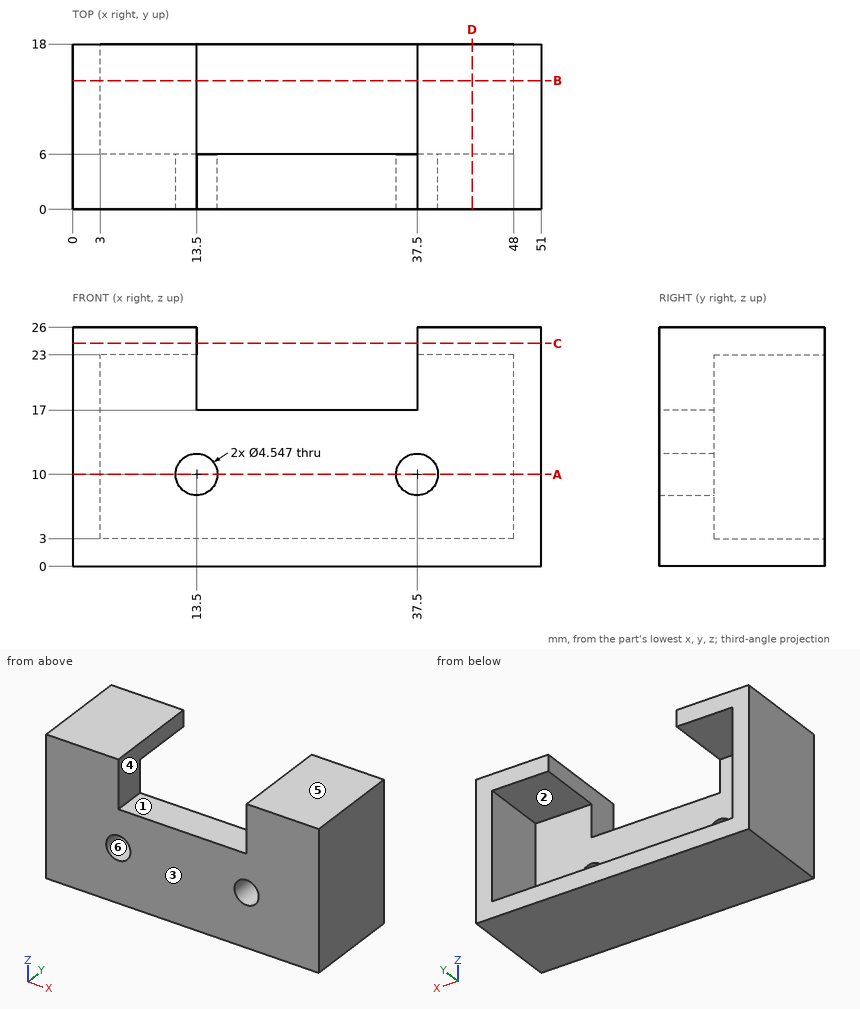
Design review of the part shown in the three views and the two pictorial views. Dimensions are in mm from the part's minimum x, y and z. A direction names the side the tool comes from. Coordinates: 2 decimals unless noted, no trailing zeros. Order: outer loops, then holes, each group sorted by start corner. A loop starts at its lowest first (then second) coordinate and runs counter-clockwise, first axis right, second up. Notation, with made-up numbers: (-6, 46) -> (7, 46) arc R24 cw to (7, 85) -> close; hole circle Ø2 at (18.25, -33). An arc over 180 degrees is marked (long way). Use one line per item in the form item = value. Start each with the question number.
(1) For probe 1 along X at (y, z) = (3.5, 10); probe 2 along X at (y, z) = (9, 8.5); probe 3 along Z at (x, y) = (10.5, 15), list the stretches that pass through material, from the lowest coordinate up.
(2) The part is to be moulded in two halves that separate along Z. For the marked faces 4, 5 and 6, say which applies: +Z half, -Z half, draft (parallel to the pull), parting line (faces both ways), or undercut.
(3) For the marked faces 1, 2 and 3, list the 3-axis set-ups (+Z, -Z, +X, -X, +Y, -Y) from which the entire face can be reached by the end or side of a thin tool; tool diameter is ignored.
(4) Add section D-D on x = 43.5. State the section outline as (y, z) points, plus the area to 3 significant figures.
(5) Insertion check: pin 1 (10 mm diameter, centred on x = 20, z = 17, fed in from +Y); pin 2 (9.5 mm diameter, centred on x = 30, y = 12.5, fed in from +Z); pin 3 (4 mm diameter, centred on x = 13.5, z = 10, fed in from +Y); pin 4 (3 mm diameter, centred on x = 29, y = 1.5, fed in from +Z). Each pin has a flat end and moves straight along its axis. Give the tip position at first contact, or say it passes through.
(6) Add section B-B on y = 14. State the section outline as (x, z) points, plus the area to 3 significant figures.
(7) Add section C-C on z = 24.25. State the section outline as (x, y) points.
(8) Add section A-A on z = 10. State the section outline as (x, y) points.
Answer block:
q1.probe_1 = 0 to 11.23, 15.77 to 35.23, 39.77 to 51
q1.probe_2 = 0 to 3, 48 to 51
q1.probe_3 = 0 to 3, 23 to 26
q2.face_4 = draft
q2.face_5 = +Z half
q2.face_6 = undercut
q3.face_1 = +Z, +Y, -Y
q3.face_2 = +Y
q3.face_3 = +Z, -Z, +X, -X, -Y
q4.outline = (0, 0) -> (18, 0) -> (18, 3) -> (6, 3) -> (6, 23) -> (18, 23) -> (18, 26) -> (0, 26) -> close
q4.area = 228 mm²
q5.pin_1 = 6
q5.pin_2 = 3
q5.pin_3 = through
q5.pin_4 = 17
q6.outline = (0, 0) -> (51, 0) -> (51, 26) -> (37.5, 26) -> (37.5, 23) -> (48, 23) -> (48, 3) -> (3, 3) -> (3, 23) -> (13.5, 23) -> (13.5, 26) -> (0, 26) -> close
q6.area = 354 mm²
q7.outline = (0, 0) -> (13.5, 0) -> (13.5, 18) -> (0, 18) -> close; (37.5, 0) -> (51, 0) -> (51, 18) -> (37.5, 18) -> close
q8.outline = (0, 0) -> (11.23, 0) -> (11.23, 6) -> (3, 6) -> (3, 18) -> (0, 18) -> close; (15.77, 0) -> (35.23, 0) -> (35.23, 6) -> (15.77, 6) -> close; (39.77, 0) -> (51, 0) -> (51, 18) -> (48, 18) -> (48, 6) -> (39.77, 6) -> close
